The model under review builds one solid part; all positions refer to its coordinate system, in mm. A direction names the side the tool comes from. Coordinates: 2 decimals unless noted, no trailing zeros. Order: outer loops, then holes, each group sorted by start corner. A loop starts at its lowest first (then second) coordinate and runs counter-clockwise, first axis right, second up.
Autodesk Inventor part; units mm, degrees
ref_plane "YZ Plane" through (0, 0, 0) normal (1, 0, 0) x (0, 1, 0)
ref_plane "XZ Plane" through (0, 0, 0) normal (0, 1, 0) x (-1, 0, 0)
ref_plane "XY Plane" through (0, 0, 0) normal (0, 0, 1) x (1, 0, 0)
sketch "Boceto1" plane through (0, 0, 0) normal (0, 0, 1) x (1, 0, 0)
  line L0 (-103, 100) -> (-103, -103)
  line L1 (-103, 100) -> (-100, 100)
  line L2 (-100, -103) -> (-100, 100)
  line L3 (-103, -103) -> (-100, -103)
  line L4 (100, 103) -> (-103, 103)
  line L5 (100, 103) -> (100, 100)
  line L6 (-103, 100) -> (100, 100)
  line L7 (-103, 103) -> (-103, 100)
  line L8 (-100, -103) -> (103, -103)
  line L9 (-100, -103) -> (-100, -100)
  line L10 (103, -100) -> (-100, -100)
  line L11 (103, -103) -> (103, -100)
  line L12 (100, -98) -> (100, 100)
  line L13 (100, 100) -> (98, 100)
  circle A0 centre (0, 0) radius 3.9
  circle A1 centre (0, 0) radius 8
  circle A2 centre (0, 0) radius 3.9
  circle A3 centre (0, 0) radius 4
  line L14 (103, 100) -> (103, -103)
  line L15 (100, -103) -> (100, 100)
  line L16 (103, -103) -> (100, -103)
  circle A4 centre (0, 0) radius 5.1
  line L17 (103, 100) -> (100, 100)
  point P0 (100, -100)
extrude "Extrusión1" add sketch "Boceto1" along normal blind 3 contours L6 L12 L15 L10 L2 | A1
sketch "Boceto2" plane through (0, 0, 3) normal (0, 0, 1) x (1, 0, 0)
  circle A0 centre (0, 0) radius 45
  line L0 (-4.4142, 5.8284) -> (-29.6244, 31.0386)
  arc A1 (-3.1395, 44.8903) -> (-29.5223, 33.9623) centre (0, 0) ccw
  line L1 (29.6244, 31.0386) -> (4.4142, 5.8284)
  arc A2 (29.5223, 33.9623) -> (3.1395, 44.8903) centre (0, 0) ccw
  arc A3 (-29.5223, 33.9623) -> (-29.6244, 31.0386) centre (-28.2102, 32.4528) ccw
  arc A4 (29.6244, 31.0386) -> (29.5223, 33.9623) centre (28.2102, 32.4528) ccw
  circle A5 centre (0, 0) radius 8
  circle A6 centre (0, 0) radius 8
  arc A7 (10.4625, 10.7488) -> (-10.4625, 10.7488) centre (0, 0) ccw
  point P0 (36.7643, -25.9497)
  point P1 (-36.7643, -25.9497)
  point P2 (-4.9054, 6.3196)
  point P3 (4.9054, 6.3196)
  point P4 (-9.8759, 11.2901)
  point P5 (9.8759, 11.2901)
extrude "Extrusión2" cut sketch "Boceto2" against normal blind 3 contours A4 L1 A7 L0 A3 A0
sketch "Boceto4" plane through (0, 0, 3) normal (0, 0, 1) x (1, 0, 0)
  circle A0 centre (0, 0) radius 55
  circle A1 centre (0, 0) radius 5.1
  line L0 (0, 0) -> (55, 0)
  circle A2 centre (55, 0) radius 1.5
  circle A3 centre (-55, 0) radius 1.5
  dimension "d14" = 55
  dimension "d15" = 3
  dimension "d16" = 3
hole "Agujero2" at (55, 0, 3) at (-55, 0, 3) direction (0, 0, -1) diameter 3 depth 4
sketch "Boceto5" plane through (0, 0, 0) normal (0, 0, -1) x (-1, 0, 0)
  circle A0 centre (88, -50) radius 2.1
  circle A1 centre (50, -88) radius 2.1
  circle A2 centre (-50, -88) radius 2.1
  circle A3 centre (-88, -50) radius 2.1
  circle A4 centre (-88, 50) radius 2.1
  circle A5 centre (-50, 88) radius 2.1
  circle A6 centre (50, 88) radius 2.1
  circle A7 centre (88, 50) radius 2.1
  point P0 (0, 0)
hole "Agujero3" at (-88, -50, 0) at (-88, 50, 0) at (-50, 88, 0) at (50, 88, 0) at (88, 50, 0) at (88, -50, 0) at (50, -88, 0) at (-50, -88, 0) direction (0, 0, 1) diameter 3 depth 4
sketch "Boceto6" plane through (0, 0, 3) normal (0, 0, 1) x (1, 0, 0)
  line L0 (20.3165, -69.168) -> (31.0665, -69.168)
  line L1 (20.3165, -74.518) -> (20.3165, -69.168)
  line L2 (-20.5835, -74.518) -> (20.3165, -74.518)
  line L3 (-20.5835, -53.818) -> (-20.5835, -74.518)
  line L4 (20.3165, -53.818) -> (-20.5835, -53.818)
  line L5 (20.3165, -59.168) -> (20.3165, -53.818)
  line L6 (31.0665, -59.168) -> (20.3165, -59.168)
  line L7 (31.0665, -43.068) -> (31.0665, -59.168)
  line L8 (23.0665, -43.068) -> (31.0665, -43.068)
  line L9 (-15.3335, -51.068) -> (15.0665, -51.068)
  line L10 (-31.3335, -43.068) -> (-23.3335, -43.068)
  line L11 (-31.3335, -85.268) -> (-31.3335, -43.068)
  line L12 (-23.3335, -85.268) -> (-31.3335, -85.268)
  line L13 (15.0665, -77.268) -> (-15.3335, -77.268)
  line L14 (31.0665, -85.268) -> (23.0665, -85.268)
  line L15 (31.0665, -69.168) -> (31.0665, -85.268)
  circle A0 centre (27.0665, -81.268) radius 2.1
  circle A1 centre (-27.3335, -81.268) radius 2.1
  circle A2 centre (27.0665, -47.068) radius 2.1
  circle A3 centre (-27.3335, -47.068) radius 2.1
  arc A4 (15.0665, -51.068) -> (23.0665, -43.068) centre (15.0665, -43.068) ccw
  arc A5 (-23.3335, -43.068) -> (-15.3335, -51.068) centre (-15.3335, -43.068) ccw
  arc A6 (-15.3335, -77.268) -> (-23.3335, -85.268) centre (-15.3335, -85.268) ccw
  arc A7 (23.0665, -85.268) -> (15.0665, -77.268) centre (15.0665, -85.268) ccw
  point P0 (0, 0)
hole "Agujero4" at (27.0665, -81.268, 3) at (27.0665, -47.068, 3) at (-27.3335, -47.068, 3) at (-27.3335, -81.268, 3) direction (0, 0, -1) diameter 3 depth 15
sketch "Boceto7" plane through (0, 0, 0) normal (0, 0, -1) x (-1, 0, 0)
  circle A0 centre (35, 95) radius 2.1
  circle A1 centre (-35, 95) radius 2.1
  circle A2 centre (35, 95) radius 1.5
  point P0 (0, 0)
  dimension "d38" = 3
hole "Agujero5" at (-35, 95, 0) at (35, 95, 0) direction (0, 0, 1) diameter 3 depth 15
sketch "Boceto8" plane through (0, 0, 0) normal (0, 0, -1) x (-1, 0, 0)
  arc A0 (-15.0665, -77.268) -> (-23.0665, -85.268) centre (-15.0665, -85.268) ccw
  line L0 (-31.0665, -85.268) -> (-23.0665, -85.268)
  line L1 (-31.0665, -69.168) -> (-31.0665, -85.268)
  line L2 (-31.0665, -43.068) -> (-31.0665, -59.168)
  line L3 (-31.0665, -59.168) -> (-20.3165, -59.168)
  line L4 (-20.3165, -69.168) -> (-31.0665, -69.168)
  line L5 (-20.0665, -54.068) -> (-20.0665, -74.268)
  line L6 (-23.0665, -43.068) -> (-31.0665, -43.068)
  line L7 (-20.3165, -69.168) -> (-40.3165, -69.168)
  line L8 (-40.3165, -69.168) -> (-40.3165, -59.168)
  line L9 (-40.3165, -59.168) -> (-20.3165, -59.168)
  line L10 (-20.3165, -59.168) -> (-20.3165, -69.168)
  point P0 (0, 0)
  dimension "d46" = 20
  dimension "d47" = 10
extrude "Extrusión3" cut sketch "Boceto8" against normal blind 10
properties part number "Soporte_Dosificador"
(1) Draft analysis for pull direction X (two halves, no side actions). For faces 3 (the face through (-24, 1, 0)), 4 (the face through (2.4, 4.5, 1.5)), state which applies: released by +X, released by -X, zero draft, split by the parting line, or undercut.
A:
face 3: zero draft
face 4: undercut
(2) We need section A-A, the plane z = 1.7. Count the separate pieces of the cut face and the enclosed holes in it, and give its area (3 significant figures).
A:
separate pieces: 1
enclosed holes: 19
area: 38,300 mm2
(3) Wall thickness on probe 1 along Y at (x, z) = (-50, 1); probe 2 along X at (y, z) = (95, 1.9); probe 3 along X at (y, z) = (-88, 2.35): over which ranges is each line inside the solid? List them lowest first.
A:
probe 1: y = -100 to -89.5, -86.5 to 86.5, 89.5 to 100
probe 2: x = -100 to -36.5, -33.5 to 33.5, 36.5 to 100
probe 3: x = -100 to -51.5, -48.5 to 48.5, 51.5 to 100
(4) We need section B-B, the plane y = 21. Write out the cut boundary in (x, z).
A:
outline: (-100, 0) - (-19.59, 0) - (-19.59, 3) - (-100, 3) - close; (19.59, 0) - (100, 0) - (100, 3) - (19.59, 3) - close
(5) We need section C-C, the plane x = -20. Write out the cut boundary in (y, z).
A:
outline: (-100, 0) - (21.41, 0) - (21.41, 3) - (-100, 3) - close; (40.31, 0) - (100, 0) - (100, 3) - (40.31, 3) - close
(6) Machinability: for faces 1 (the face through (-24, 1, 3)), 2 (the face through (-19.612, 21.026, 1.521)), which of the approach directions +Z, -Z, +X, -X, +Y, -Y give a long, thin tool a straight path to every point of the face, cutting with its end or side? Answer none if there is none.
A:
face 1: +Z, +X, -X, +Y, -Y
face 2: +Z, -Z
